Build history of the part. All positions in model axes, mm. Face numbers are marked on the shaded views. A direction names the side the tool comes from. Round coordinates to 2 decimals unless told otherwise and drop trailing zeros. Loops run counter-clockwise (first coordinate to the right, second up) from the corner with the lowest first, then second, coordinate; pieces in that order, holes last. Notation, with made-up numbers: (-19.75, -4) -> (-12.75, -4) arc R25 ccw to (-12.75, 14) -> close; hole circle Ø6 at (11.5, 20). An arc over 180 degrees is marked (long way). Put each result on its own line as item: value. Start each with the question number.
Item 1: Cut at A-A, the plane y = 10. List the corners of the cut face in (x, z) (3 decimals), plus the area to 3 significant figures.
Item 2: Cut at C-C, the plane z = -51. List the corners of the cut face in (x, y).
Item 3: Pull direction Z, two halves, no side cores. Call the marked faces 3, 4 and 5: +Z half, -Z half, draft (parallel to the pull), parting line (faces both ways), or undercut.
Item 4: Drill centre lines: probe 1 along Z at (x, y) = (-269, 7.75); probe 2 along Z at (x, y) = (-260, 2.25); probe 3 along X at (y, z) = (5.5, -6). Where is each one in solid material? Low to high. Write a range as [from, to].
Item 5: Cut at B-B, the plane x = -265. List the corners of the cut face in (y, z).
Item 6: Tool access for the marked faces 1 and 2: list every direction of +Z, -Z, +X, -X, +Y, -Y with a clear straight run to the whole face (end or side of a thin tool).
Item 7: Flat gauge pins, fed straight in: pin 1 Ø5 at (y, z) = (5.5, -62.5) entering from -X; pin 2 Ø3 at (x, y) = (-265, 5) entering from -Z. Where does each tip first touch, or does it go through?
Item 8: Cut at D-D, the plane x = -247.5. List the corners of the cut face in (y, z), plus the area to 3 significant figures.
```python
from build123d import *

# Parameters (mm, degrees)
BOSS_EXTRUDE1_DEPTH = 12


with BuildPart() as part:
    # Sketch1 → Boss-Extrude1 (new body)
    with BuildSketch(Plane(origin=(0, 0, 0), x_dir=(1, 0, 0), z_dir=(0, 1, 0))):
        with BuildLine():
            Line((-272.719864834, 112.964266743), (-235.764662876, 97.656920891))
            ThreePointArc((-235.764662876, 97.656920891), (-250.286431131, 49.785066539), (-255.189832201, 0))
            Line((-255.189832201, 0), (-295.127762341, 0))
            Line((-295.127762341, 0), (-295.127762341, 6.054265565))
            ThreePointArc((-295.127762341, 6.054265565), (-288.912043726, 60.55477872), (-272.719864834, 112.964266743))
        make_face()
        Polygon((-249.614999445, 73.084292156), (-254.615566779, 52.688353189), (-284.723857635, 60.070143062), (-279.723290301, 80.466082029), align=None, mode=Mode.SUBTRACT)
        Polygon((-241.658318908, 96.615135023), (-248.580348619, 76.788750968), (-277.847867938, 87.006985303), (-270.925838227, 106.833369358), align=None, mode=Mode.SUBTRACT)
        Polygon((-255.292380187, 48.902135943), (-258.325942442, 28.122398215), (-289.000793374, 32.600513925), (-285.967231118, 53.380251653), align=None, mode=Mode.SUBTRACT)
        Polygon((-258.638754349, 24.288905534), (-259.677683338, 3.314620647), (-290.639722934, 4.848277725), (-289.600793945, 25.822562613), align=None, mode=Mode.SUBTRACT)
    extrude(amount=BOSS_EXTRUDE1_DEPTH)


solid = part.part
```
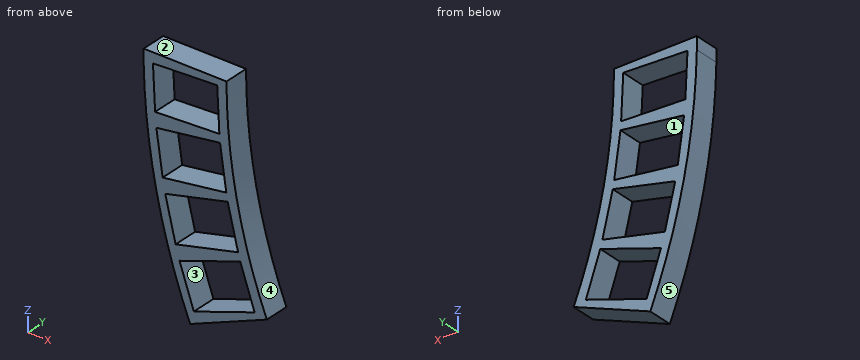
Reply:
1. outline: (-295.128, -6.054) arc R295.19 ccw to (-272.72, -112.964) -> (-235.765, -97.657) arc R255.19 cw to (-255.19, 0) -> (-295.128, 0) -> close; hole (-290.64, -4.848) -> (-289.601, -25.823) -> (-258.639, -24.289) -> (-259.678, -3.315) -> close; hole (-289.001, -32.601) -> (-285.967, -53.38) -> (-255.292, -48.902) -> (-258.326, -28.122) -> close; hole (-284.724, -60.07) -> (-279.723, -80.466) -> (-249.615, -73.084) -> (-254.616, -52.688) -> close; hole (-277.848, -87.007) -> (-270.926, -106.833) -> (-241.658, -96.615) -> (-248.58, -76.789) -> close
1. area: 1,720 mm^2
2. outline: (-290.75, 0) -> (-286.31, 0) -> (-286.31, 12) -> (-290.75, 12) -> close; (-269.66, 0) -> (-250.04, 0) -> (-250.04, 12) -> (-269.66, 12) -> close
3. face 3: undercut
3. face 4: +Z half
3. face 5: -Z half
4. probe 1: z = [-111.42, -106.16], [-83.92, -77.84], [-56.22, -50.9], [-29.68, -24.8], [-3.78, 0]
4. probe 2: z = [-107.7, -103.02], [-80.78, -75.63], [-54.01, -49.59], [-28.37, -24.36], [-3.33, 0]
4. probe 3: x = [-295.13, -290.58], [-259.54, -255.12]
5. outline: (0, -109.77) -> (12, -109.77) -> (12, -104.76) -> (0, -104.76) -> close; (0, -82.52) -> (12, -82.52) -> (12, -76.86) -> (0, -76.86) -> close; (0, -55.23) -> (12, -55.23) -> (12, -50.32) -> (0, -50.32) -> close; (0, -29.1) -> (12, -29.1) -> (12, -24.6) -> (0, -24.6) -> close; (0, -3.58) -> (12, -3.58) -> (12, 0) -> (0, 0) -> close
6. face 1: +Y, -Y
6. face 2: +Z, +X, -X, +Y, -Y
7. pin 1: stops at x = -289.03
7. pin 2: stops at z = -110.39
8. outline: (0, -102.52) -> (12, -102.52) -> (12, -98.65) -> (0, -98.65) -> close; (0, -79.88) -> (12, -79.88) -> (12, -62.17) -> (0, -62.17) -> close
8. area: 259 mm^2
